Part model, mm, in its own coordinate system. Face numbers are marked on the shaded views. A direction names the side the tool comes from. Round coordinates to 2 decimals unless told otherwise and drop trailing zeros. Order: outer loops, then holes, each group sorted by start corner. A loop starts at its lowest first (then second) coordinate and runs counter-clockwise, first axis right, second up. Notation, with made-up numbers: (19, -8.5) -> (55, -8.5) arc R4 ccw to (55, -4.5) -> close; hole circle Ø10 at (-17, -22.5). An arc over 180 degrees is marked (long way). Return JSON: item names as keys, results as strings. Group by question number.
from build123d import *

# Parameters (mm, degrees)
SKETCH1_W           = 13.2
SKETCH1_H           = 19.2
BOSS_EXTRUDE1_DEPTH = 11.7
SKETCH2_W           = 15
SKETCH2_H           = 21
BOSS_EXTRUDE2_DEPTH = 1.5
SKETCH3_W           = 13.2
SKETCH3_H           = 19.2
BOSS_EXTRUDE3_DEPTH = 5
CUT_EXTRUDE1_DEPTH  = 13.2
SKETCH5_W           = 4.8
SKETCH5_H           = 1
BOSS_EXTRUDE4_DEPTH = 8.2
FILLET1_R           = 1


with BuildPart() as part:
    # Sketch1 → Boss-Extrude1 (new body)
    with BuildSketch(Plane(origin=(0, 0, 0), x_dir=(1, 0, 0), z_dir=(0, 1, 0))):
        Rectangle(SKETCH1_W, SKETCH1_H)
    extrude(amount=BOSS_EXTRUDE1_DEPTH)

    # Sketch2 → Boss-Extrude2 (add)
    with BuildSketch(Plane(origin=(0, 11.7, 0), x_dir=(1, 0, 0), z_dir=(0, 1, 0))):
        Rectangle(SKETCH2_W, SKETCH2_H)
    extrude(amount=BOSS_EXTRUDE2_DEPTH)

    # Sketch3 → Boss-Extrude3 (add)
    with BuildSketch(Plane(origin=(0, 13.2, 0), x_dir=(1, 0, 0), z_dir=(0, 1, 0))):
        Rectangle(SKETCH3_W, SKETCH3_H)
    extrude(amount=BOSS_EXTRUDE3_DEPTH)

    # Sketch4 → Cut-Extrude1 (cut)
    with BuildSketch(Plane(origin=(6.6, 0, 0), x_dir=(0, 0, -1), z_dir=(1, 0, 0))):
        Polygon((-9.6, 18.2), (-9.6, 15.7), (-9.6, 14.2), (9.6, 15.2), (9.6, 18.2), align=None)
    extrude(amount=-CUT_EXTRUDE1_DEPTH, mode=Mode.SUBTRACT)

    # Sketch5 → Boss-Extrude4 (add)
    with BuildSketch(Plane.XZ):
        with Locations((0, 1.5)):
            Rectangle(SKETCH5_W, SKETCH5_H)
        with Locations((0, 7.6)):
            Rectangle(SKETCH5_W, SKETCH5_H)
    extrude(amount=BOSS_EXTRUDE4_DEPTH)

    # Fillet1
    fillet1_edges = [part.edges().sort_by_distance(p)[0] for p in [
        (7.5, 12.45, 10.5),
        (7.5, 12.45, -10.5),
        (-7.5, 12.45, -10.5),
        (-7.5, 12.45, 10.5),
        (0, 15.2, -9.6),
        (0, 14.2, 9.6),
    ]]
    fillet(fillet1_edges, radius=FILLET1_R)


solid = part.part
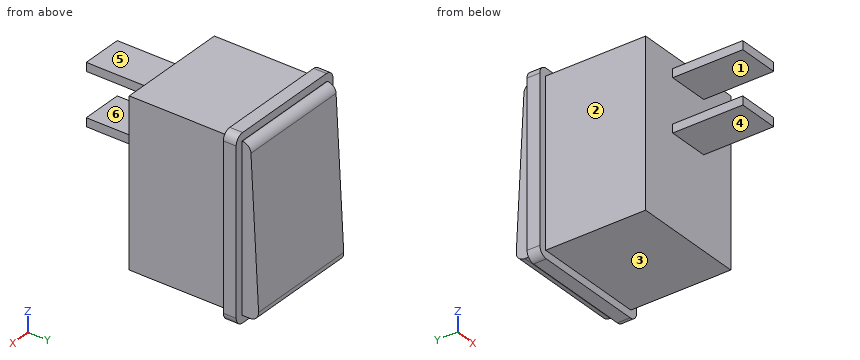
(1) Saw through at D-D, the plane z = 7.5. List the corners of the cut face in (x, y).
(2) Saw through at B-B, the plane z = 3.5. List the corners of the cut face in (x, y), and give its area (3 significant figures).
(3) Probe L1, parallel to Z at x = -3.25, y = 10.25; L2, parallel to X at y = 10.5, z = 9; L3, parallel to Y at x = 4.5, z = -4.25. List the from-to ranges inside material, lowest first. Write a range as [from, to].
(4) Saw through at A-A, the plane x = 3.5. List the corners of the cut face in (y, z), and give its area (3 significant figures).
(5) Tool access for the marked faces 4, 5 and 6: list every direction of +Z, -Z, +X, -X, +Y, -Y with a clear straight run to the whole face (end or side of a thin tool).
(6) Saw through at C-C, the plane y = 4.25. List the corners of the cut face in (x, z), and give its area (3 significant figures).
(7) Mould opens along Z. For the marked faces 1, 2 and 3 say: pulls with the +Z half, pulls with the -Z half, needs draft (parallel to the pull), parting line crosses it, or undercut.
(8) Pin check, flat tips, straight feed: P1, Ø4, axis at y = -4.5, z = -0.5, coming from the +X side; P2, Ø5.5, axis at x = 1, y = -3, coming from the -Z side; P3, Ø0.8, axis at y = -5.5, z = 7.5, coming from the -X side; P4, Ø1, axis at x = -3, y = -4, coming from the -Z side. Stop position of each tip, or through.
Results are:
{
 "1": {"outline": "(-7.5, 11.7) -> (-6.6, 11.7) -> (-6.6, 0) -> (-2.4, 0) -> (-2.4, -8.2) -> (2.4, -8.2) -> (2.4, 0) -> (6.6, 0) -> (6.6, 11.7) -> (7.5, 11.7) -> (7.5, 13.2) -> (6.6, 13.2) -> (6.6, 14.31) -> (-6.6, 14.31) -> (-6.6, 13.2) -> (-7.5, 13.2) -> close"},
 "2": {"outline": "(-7.5, 11.7) -> (-6.6, 11.7) -> (-6.6, 0) -> (6.6, 0) -> (6.6, 11.7) -> (7.5, 11.7) -> (7.5, 13.2) -> (6.6, 13.2) -> (6.6, 14.52) -> (-6.6, 14.52) -> (-6.6, 13.2) -> (-7.5, 13.2) -> close", "area": "194 mm^2"},
 "3": {"L1": "z = [-9.6, 9.6]", "L2": "x = [-6.6, 6.6]", "L3": "y = [0, 14.92]"},
 "4": {"outline": "(0, -9.6) -> (11.7, -9.6) -> (11.7, -10.5) -> (13.2, -10.5) -> (13.2, -9.6) -> (14.15, -9.6) arc R1 ccw to (15.15, -8.55) -> (14.25, 8.65) arc R1 ccw to (13.25, 9.6) -> (13.2, 9.6) -> (13.2, 10.5) -> (11.7, 10.5) -> (11.7, 9.6) -> (0, 9.6) -> close", "area": "285 mm^2"},
 "5": {"face 4": "-Z, +X, -X, -Y", "face 5": "+Z, +X, -X, -Y", "face 6": "+X, -X, -Y"},
 "6": {"outline": "(-6.6, -9.6) -> (6.6, -9.6) -> (6.6, 9.6) -> (-6.6, 9.6) -> close", "area": "253 mm^2"},
 "7": {"face 1": "undercut", "face 2": "needs draft", "face 3": "pulls with the -Z half"},
 "8": {"P1": "stops at x = 2.4", "P2": "stops at z = 1", "P3": "stops at x = -2.4", "P4": "passes through"}
}
